CAD build for the part. Positions are in the model's coordinates, mm. Face numbers are marked on the shaded views. Round coordinates to 2 decimals unless told otherwise and drop trailing zeros. Loops run counter-clockwise (first coordinate to the right, second up) from the corner with the lowest first, then second, coordinate; pieces in that order, holes last.
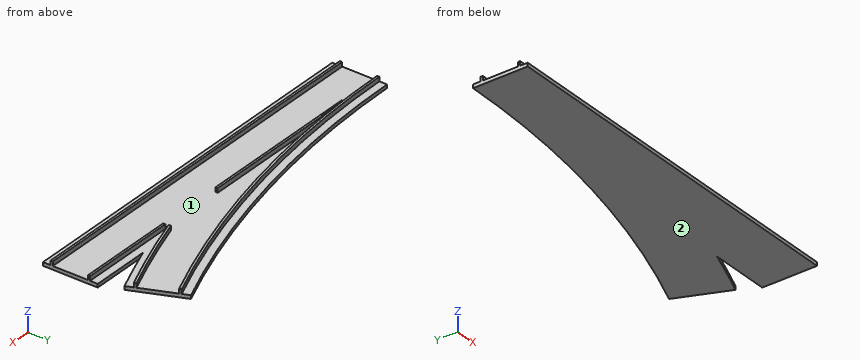
from build123d import *

# Parameters (mm, degrees)
PAD_DEPTH     = 1.6
SKETCH001_W   = 174
SKETCH001_H   = 1
SKETCH001_W_2 = 45.298462
PAD001_DEPTH  = 2


with BuildPart() as part:
    # Sketch → Pad (new body)
    with BuildSketch(Plane.XY):
        with BuildLine():
            Line((0, -12.5), (174, -12.5))
            Line((174, -12.5), (174, 12.5))
            Line((174, 12.5), (146.628783, 12.5))
            ThreePointArc((146.628783, 12.5), (158.042748, 16.685665), (169.337419, 21.183307))
            Line((159.770333, 44.280295), (169.337419, 21.183307))
            ThreePointArc((0, 12.5), (81.450209, 20.522145), (159.770333, 44.280295))
            Line((0, -12.5), (0, 12.5))
        make_face()
    extrude(amount=PAD_DEPTH)

    # Sketch001 (on Face9 of Pad) → Pad001 (join)
    with BuildSketch(Plane.XY.offset(1.6)):
        with Locations((87, -8.5)):
            Rectangle(SKETCH001_W, SKETCH001_H)
        with BuildLine():
            ThreePointArc((0, 8), (82.328116, 16.108612), (161.492408, 40.122837))
            Line((161.109725, 41.046717), (161.492408, 40.122837))
            ThreePointArc((0, 9), (82.133026, 17.089397), (161.109725, 41.046717))
            Line((0, 9), (0, 8))
        make_face()
        with BuildLine():
            ThreePointArc((128.49115, 10.225031), (148.414319, 16.848466), (167.998027, 24.416885))
            Line((167.615343, 25.340765), (167.998027, 24.416885))
            ThreePointArc((128.198459, 11.181238), (148.076245, 17.789586), (167.615343, 25.340765))
            Line((128.198459, 11.181238), (128.49115, 10.225031))
        make_face()
        with Locations((151.350769, 8.5)):
            Rectangle(SKETCH001_W_2, SKETCH001_H)
        with BuildLine():
            Line((97.217995, 8), (97.217995, 9))
            Line((97.217995, 9), (35.878481, 9))
            ThreePointArc((21.077604, 8), (28.482431, 8.435039), (35.878481, 9))
            Line((97.217995, 8), (21.077604, 8))
        make_face()
    extrude(amount=PAD001_DEPTH)


solid = part.part
Item 1: Wall check: L1, parallel to Y at x = 82, z = 2.4; L2, parallel to Y at x = 96, z = 2.35; L3, parallel to Y at x = 141, z = 3.5. Give the ranges that are in metal, low to high.
Verdict:
L1: y = -9 to -8, 8 to 9, 16.04 to 17.06
L2: y = -9 to -8, 8 to 9, 19.06 to 20.09
L3: y = -9 to -8, 8 to 9, 14.26 to 15.32, 32.25 to 33.31
Item 2: Cut at A-A (z = 2.8). List the corners of the cut face in (x, y), plus the area to 3 significant figures.
Verdict:
outline: (0, -9) - (174, -9) - (174, -8) - (0, -8) - close; (0, 8) arc R422 ccw to (161.49, 40.12) - (161.11, 41.05) arc R421 cw to (0, 9) - close; (21.08, 8) - (97.22, 8) - (97.22, 9) - (35.88, 9) arc R422.53 cw to start; (128.2, 11.18) - (128.49, 10.23) arc R439 ccw to (168, 24.42) - (167.62, 25.34) arc R438 cw to start; (128.7, 8) - (174, 8) - (174, 9) - (128.7, 9) - close
area: 495 mm2
Item 3: Mould opens along X. For the marked faces 1 and 2 say: released by +X, released by -X, zero draft, split by the parting line, or undercut.
Verdict:
face 1: undercut
face 2: zero draft
Item 4: Cut at D-D (x = 46.5). List the corners of the cut face in (y, z), plus the area to 3 significant figures.
Verdict:
outline: (-12.5, 0) - (15.1, 0) - (15.1, 1.6) - (11.58, 1.6) - (11.58, 3.6) - (10.57, 3.6) - (10.57, 1.6) - (9, 1.6) - (9, 3.6) - (8, 3.6) - (8, 1.6) - (-8, 1.6) - (-8, 3.6) - (-9, 3.6) - (-9, 1.6) - (-12.5, 1.6) - close
area: 50.2 mm2
Item 5: Cut at B-B (x = 16). List the corners of the cut face in (y, z).
Verdict:
outline: (-12.5, 0) - (12.81, 0) - (12.81, 1.6) - (9.3, 1.6) - (9.3, 3.6) - (8.3, 3.6) - (8.3, 1.6) - (-8, 1.6) - (-8, 3.6) - (-9, 3.6) - (-9, 1.6) - (-12.5, 1.6) - close
Item 6: Flat gauge pins, fed straight in: P1, Ø1.6, axis at x = 53.5, z = 3, coming from the -Y side; P2, Ø1.6, axis at x = 115.5, z = 2.5, coming from the +Y side; P3, Ø3, axis at x = 91.5, y = 12.5, coming from the +Z side. Where does each tip first touch, or does it go through?
Verdict:
P1: stops at y = -9
P2: stops at y = 25.38
P3: stops at z = 1.6
Item 7: Cut at C-C (y = 27.5). List the corners of the cut face in (x, z).
Verdict:
outline: (110.91, 0) - (166.72, 0) - (166.72, 1.6) - (126.8, 1.6) - (126.8, 3.6) - (123.43, 3.6) - (123.43, 1.6) - (110.91, 1.6) - close
